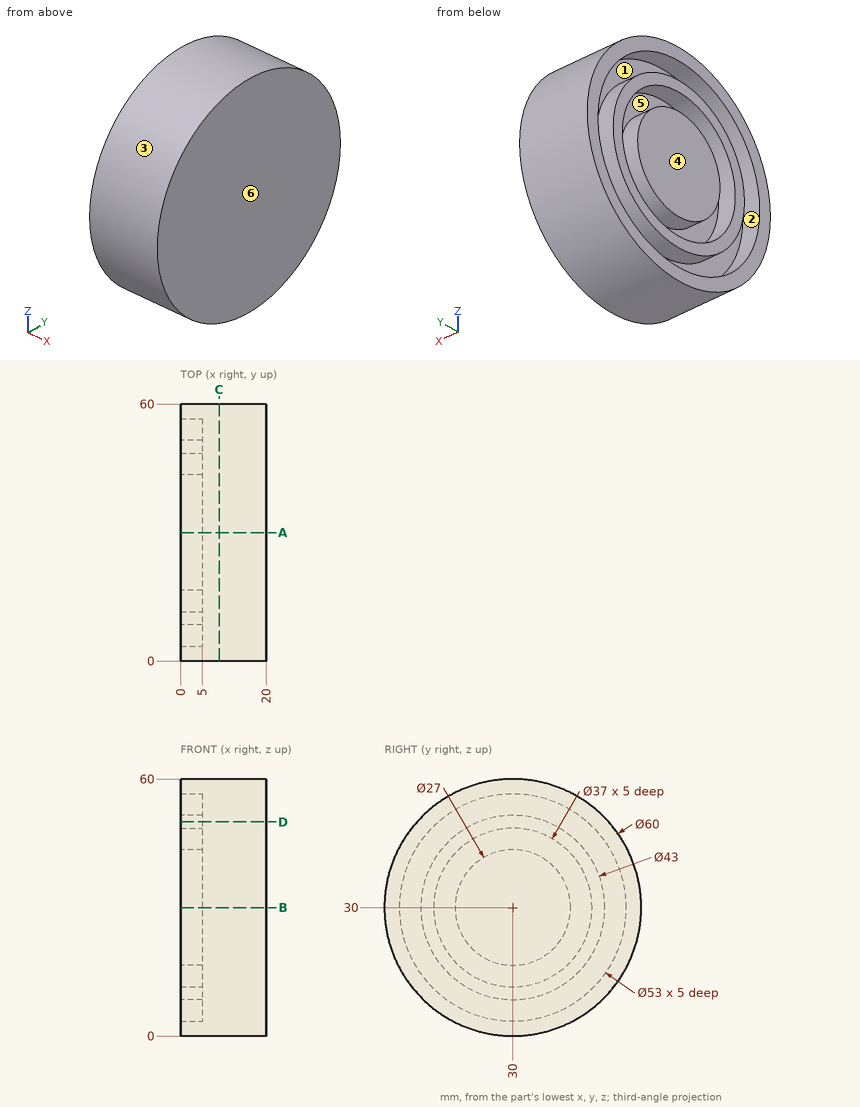
Geometry: see drawing. Coordinates: mm, zero at the bounding-box minimum. A direction names the side the tool comes from. Coordinates: 2 decimals unless noted, no trailing zeros. Order: outer loops, then holes, each group sorted by start corner. A loop starts at its lowest first (then second) coordinate and runs counter-clockwise, first axis right, second up. Notation, with made-up numbers: (80.25, 31.25) -> (101.25, 31.25) arc R21 ccw to (101.25, 63.25) -> close; hole circle Ø10 at (-12.75, -14.5). An arc over 180 degrees is marked (long way). Write each question's results on one line, items separated by ' | '. Start each with the question number.
1) Cut plane D-D, the plane z = 50. Output: boundary loops of the cut face in (x, y).
2) Mould query, pull axis Y, two halves, no side actions, for the marked faces 1, 2, 3 and 4. Classes: released by +Y, released by -Y, zero draft, split by the parting line, or undercut.
3) Cut plane A-A, the plane y = 30. Output: boundary loops of the cut face in (x, z).
4) First-contact query: pin 1 (12 mm diameter, centred on x = 15, z = 8.5, fed in from -Y); pin 2 (4 mm diameter, centred on x = 5, y = 32, fed in from +Z); pin 3 (1 mm diameter, centred on x = 9.5, z = 49.5, fed in from +Y). Flat tips, straight axial feed; report the tip coordinate or a pass-through.
5) Material intervals for line 1 along Z through (x, y) = (3.2, 30); line 2 along Y through (x, z) = (1.5, 41.5); line 3 along X through (y, z) = (27, 4), sorted ascending.
6) Set-up query: the marked faces 5 and 6. Return all of +Z, -Z, +X, -X, +Y, -Y with unobstructed straight access to the full face (end or side cutting, diameter ignored); none if empty.
7) Cut plane C-C, the plane x = 9. Output: boundary loops of the cut face in (y, z), and give its area (3 significant figures).
Checks:
1) outline: (0, 7.64) -> (20, 7.64) -> (20, 52.36) -> (0, 52.36) -> (0, 47.39) -> (5, 47.39) -> (5, 37.89) -> (0, 37.89) -> (0, 22.11) -> (5, 22.11) -> (5, 12.61) -> (0, 12.61) -> close
2) face 1: undercut | face 2: undercut | face 3: split by the parting line | face 4: zero draft
3) outline: (0, 0) -> (20, 0) -> (20, 60) -> (0, 60) -> (0, 56.5) -> (5, 56.5) -> (5, 51.5) -> (0, 51.5) -> (0, 48.5) -> (5, 48.5) -> (5, 43.5) -> (0, 43.5) -> (0, 16.5) -> (5, 16.5) -> (5, 11.5) -> (0, 11.5) -> (0, 8.5) -> (5, 8.5) -> (5, 3.5) -> (0, 3.5) -> close
4) pin 1: y = 4.31 | pin 2: z = 60 | pin 3: y = 53.22
5) line 1: 0 to 3.5, 8.5 to 11.5, 16.5 to 43.5, 48.5 to 51.5, 56.5 to 60 | line 2: 2.29 to 6.13, 11.83 to 15.51, 22.93 to 37.07, 44.49 to 48.17, 53.87 to 57.71 | line 3: 5 to 20
6) face 5: -X | face 6: +Z, -Z, +X, +Y, -Y
7) outline: circle Ø60 at (30, 30) | area: 2,830 mm^2
